Build history of the part. All positions in model axes, mm. A direction names the side the tool comes from. Give positions to 0.01 mm unless a question says otherwise; leave off trailing zeros. Loops run counter-clockwise (first coordinate to the right, second up) from the corner with the lowest first, then second, coordinate; pieces in that order, holes last.
1) Flat gauge pins, fed straight in: P1, Ø1.5, axis at y = -21.5, z = 154.5, coming from the +X side; P2, Ø8, axis at x = 126.5, z = 220.5, coming from the -Y side; P3, Ø8, axis at x = 128, z = 122, coming from the -Y side. Where does each tip first touch, or does it go through?
2) Band-saw the part on C-C on y = -3. List the corners of the cut face in (x, z).
3) Wall check: line 1 (Z direction, x = 153.5, y = 54.5); line 2 (Y direction, x = 149, z = 31.5); line 3 (Y direction, x = 136, z = 15.5). Give the ranges that are in metal, low to high.
4) Two-plate mould, pull along Y, no slides. Class faces 1 (the flat face through (161, 14, 0)), 2 (the cylindrical face through (153.66, 57.33, 11.85)), 3 (the cylindrical face through (123.97, 95.7, 3.01)), 4 (the flat face through (157.261, -57.084, 121.278)): +Y half, -Y half, draft (parallel to the pull), parting line (faces both ways), or undercut.
5) Band-saw the part on A-A on z = 203.5. List the corners of the cut face in (x, y).
6) Band-saw the part on D-D on x = 133. List the corners of the cut face in (y, z).
7) Band-saw the part on B-B on x = 161.5. List the corners of the cut face in (y, z).
8) 3-axis set-ups, long thin cutter, end or side, ignore diameter. For faces 5 (the cylindrical face through (166.364, -14.721, 235.974)), 6 (the flat face through (135, 87.07, 121.28)): which of +Z, -Z, +X, -X, +Y, -Y reach the whole face in a straight line?
```python
from build123d import *

# Parameters (mm, degrees)
BASE_FLANGE1_DEPTH = 246
FILLET1_START      = -79
FILLET1_DEPTH      = 4
FILLET1_START_2    = 148
FILLET1_2_DEPTH    = 3
SKETCH6_R          = 3
CUT_EXTRUDE1_DEPTH = 1.5


with BuildPart() as part:
    # Base-Flange1: sheet metal written as solids
    # Sketch1 → Base-Flange1 (new body)
    with BuildSketch(Plane.XY):
        with BuildLine():
            Line((135.953063945, -76.256345678), (140.443766564, -76.256345678))
            ThreePointArc((140.443766564, -76.256345678), (141.829012404, -75.917378177), (142.901222697, -74.977074987))
            Line((142.901222697, -74.977074987), (168.801582917, -37.987527165))
            ThreePointArc((168.801582917, -37.987527165), (169.273014805, -36.916116698), (169.298550043, -35.745853323))
            Line((169.298550043, -35.745853323), (169.167035978, -35))
            Line((169.167035978, -35), (149.639554036, 75.745853323))
            ThreePointArc((149.639554036, 75.745853323), (149.215305114, 76.836807615), (148.405860086, 77.682364923))
            Line((148.405860086, 77.682364923), (121.208107966, 96.72643598))
            Line((121.208107966, 96.72643598), (122.06847262, 97.955164046))
            Line((122.06847262, 97.955164046), (149.266224741, 78.911092989))
            ThreePointArc((149.266224741, 78.911092989), (150.480392283, 77.642757028), (151.116765666, 76.00632559))
            Line((151.116765666, 76.00632559), (170.644247608, -34.739527733))
            Line((170.644247608, -34.739527733), (170.775761672, -35.485381057))
            ThreePointArc((170.775761672, -35.485381057), (170.737458816, -37.240776119), (170.030310983, -38.84789182))
            Line((170.030310983, -38.84789182), (144.129950763, -75.837439642))
            ThreePointArc((144.129950763, -75.837439642), (142.521635324, -77.247894427), (140.443766564, -77.756345678))
            Line((140.443766564, -77.756345678), (135.953063945, -77.756345678))
            Line((135.953063945, -77.756345678), (135.953063945, -76.256345678))
        make_face()
    extrude(amount=BASE_FLANGE1_DEPTH)

    # Fillet1: read off the stored shape, not the designer's step
    # Fillet1 outline → Fillet1 (cut)
    with BuildSketch(Plane(origin=(0, 0, 0), x_dir=(1, 0, 0), z_dir=(0, 1, 0)).offset(FILLET1_START)):
        with BuildLine():
            Line((135.953063945, 0), (135.953063945, -8.345516304))
            ThreePointArc((135.953063945, -8.345516304), (137.147015631, -3.607002497), (140.443766564, 0))
            Line((140.443766564, 0), (135.953063945, 0))
        make_face()
        with BuildLine():
            ThreePointArc((140.443766564, -246), (137.147015631, -242.392997503), (135.953063945, -237.654483696))
            Line((135.953063945, -237.654483696), (135.953063945, -246))
            Line((135.953063945, -246), (140.443766564, -246))
        make_face()
    extrude(amount=FILLET1_DEPTH, mode=Mode.SUBTRACT)

    # Fillet1 2 outline → Fillet1 2 (cut)
    with BuildSketch(Plane(origin=(0, 0, 0), x_dir=(0.819152044288989, -0.5735764363510502, 0), z_dir=(0.57357643635105, 0.819152044288989, 0)).offset(FILLET1_START_2)):
        with BuildLine():
            Line((43.807864974, 0), (43.807864974, -10))
            ThreePointArc((43.807864974, -10), (46.736797162, -2.928932188), (53.807864974, 0))
            Line((53.807864974, 0), (43.807864974, 0))
        make_face()
        with BuildLine():
            ThreePointArc((53.807864974, -246), (46.736797162, -243.071067812), (43.807864974, -236))
            Line((43.807864974, -236), (43.807864974, -246))
            Line((43.807864974, -246), (53.807864974, -246))
        make_face()
    extrude(amount=FILLET1_2_DEPTH, mode=Mode.SUBTRACT)

    # Sketch6 → Cut-Extrude1 (cut)
    with BuildSketch(Plane(origin=(159.557884805, 28.134360076, 0), x_dir=(0, 0, -1), z_dir=(0.984807753012208, 0.17364817766693147, 0))):
        with Locations(Location((-233, 27.004644779, 0), (0, 0, 90))):
            Circle(SKETCH6_R)
        with Locations(Location((-233, -42.995355221, 0), (0, 0, 90))):
            Circle(SKETCH6_R)
        with Locations(Location((-13, -42.995355221, 0), (0, 0, 90))):
            Circle(SKETCH6_R)
        with Locations(Location((-13, 27.004644779, 0), (0, 0, 90))):
            Circle(SKETCH6_R)
    extrude(amount=-CUT_EXTRUDE1_DEPTH, mode=Mode.SUBTRACT)


solid = part.part
```
Findings below:
1. P1: stops at x = 168.44
1. P2: stops at y = 90.22
1. P3: stops at y = 89.17
2. outline: (163.52, 0) - (165.05, 0) - (165.05, 246) - (163.52, 246) - close
3. line 1: z = 0 to 10, 16 to 230, 236 to 246
3. line 2: y = -68.88 to -66.27, 77.13 to 79.1
3. line 3: y = -77.76 to -76.26, 86.37 to 88.2
4. face 1: draft
4. face 2: undercut
4. face 3: +Y half
4. face 4: -Y half
5. outline: (121.21, 96.73) - (148.41, 77.68) arc R3 cw to (149.64, 75.75) - (169.3, -35.75) arc R3 cw to (168.8, -37.99) - (142.9, -74.98) arc R3 cw to (140.44, -76.26) - (135.95, -76.26) - (135.95, -77.76) - (140.44, -77.76) arc R4.5 ccw to (144.13, -75.84) - (170.03, -38.85) arc R4.5 ccw to (170.78, -35.49) - (151.12, 76.01) arc R4.5 ccw to (149.27, 78.91) - (122.07, 97.96) - close
6. outline: (88.47, 0) - (90.3, 0) - (90.3, 246) - (88.47, 246) - close
7. outline: (-51.03, 0) - (-48.42, 0) - (-48.42, 246) - (-51.03, 246) - close; (8.48, 0) - (17.12, 0) - (17.12, 246) - (8.48, 246) - close
8. face 5: none
8. face 6: +Z, -Z, -X
